Autodesk Fusion 360 part; units mm, degrees
sketch "Sketch1" plane through (0, 0, 0) normal (0, 0, 1) x (1, 0, 0)
  line L0 (0, 0) -> (26, 0)
  line L1 (26, 0) -> (26, 35.8)
  line L2 (26, 35.8) -> (0, 35.8)
  line L3 (0, 35.8) -> (0, 0)
  circle A0 centre (23.75, 30.8) radius 1.5
  circle A1 centre (2.25, 30.8) radius 1.5
  circle A2 centre (2.25, 4.8) radius 1.5
  circle A3 centre (23.75, 4.8) radius 1.5
  circle A4 centre (13, 25.8) radius 3.5
  line L4 (21.5, 27.2) -> (20.2, 27.2)
  line L5 (20.2, 27.2) -> (20.2, 24.4)
  line L6 (20.2, 24.4) -> (21.5, 24.4)
  line L7 (21.5, 24.4) -> (21.5, 27.2)
  dimension "d1" = 26
  dimension "d2" = 35.8
  dimension "d3" = 3
  dimension "d4" = 3
  dimension "d5" = 3
  dimension "d6" = 3
  dimension "d7" = 5
  dimension "d10" = 31
  dimension "d11" = 31
  dimension "d12" = 5
  dimension "d13" = 2.25
  dimension "d14" = 2.25
  dimension "d15" = 2.25
  dimension "d16" = 2.25
  dimension "d17" = 7
  dimension "d18" = 10
  dimension "d21" = 1.3
  dimension "d22" = 2.8
  dimension "d23" = 13
  dimension "d24" = 7.2
  dimension "d25" = 8.6
extrude "Extrude1" add sketch "Sketch1" along normal blind 2
Read the model definition and answer for the solid it produces. Units are mm, in the model's axes. A direction names the side the tool comes from. Coordinates: 2 decimals unless noted, no trailing zeros. Order: outer loops, then holes, each group sorted by start corner. A loop starts at its lowest first (then second) coordinate and runs counter-clockwise, first axis right, second up. Notation, with made-up numbers: (5.5, -21.75) -> (32.5, -21.75) arc R33 cw to (32.5, 9.25) -> close; hole circle Ø1 at (66, 1). An arc over 180 degrees is marked (long way). Answer as a JSON object with one key per item and string values.
1) The mould has two halves that part along Y. Classify faces 1 (the face through (1.925, 32.264, 0.986)), 2 (the face through (13, 35.8, 1)), 3 (the face through (23.425, 32.264, 0.986)), 4 (the face through (0, 18, 1)): released by +Y, released by -Y, zero draft, split by the parting line, or undercut.
Model answer:
{"face 1": "undercut", "face 2": "released by +Y", "face 3": "undercut", "face 4": "zero draft"}
2) A cutting plane is placed at A-A, the plane y = 4.8. Determine the outline of the cut face in (x, z).
Model answer:
{"outline": "(0, 0) -> (0.75, 0) -> (0.75, 2) -> (0, 2) -> close; (3.75, 0) -> (22.25, 0) -> (22.25, 2) -> (3.75, 2) -> close; (25.25, 0) -> (26, 0) -> (26, 2) -> (25.25, 2) -> close"}
3) A cutting plane is placed at D-D, the plane x = 13. Determine the outline of the cut face in (y, z), plus the area to 3 significant figures.
Model answer:
{"outline": "(0, 0) -> (22.3, 0) -> (22.3, 2) -> (0, 2) -> close; (29.3, 0) -> (35.8, 0) -> (35.8, 2) -> (29.3, 2) -> close", "area": "57.6 mm²"}
4) A cutting plane is placed at C-C, the plane z = 0.5. Determine the outline of the cut face in (x, y).
Model answer:
{"outline": "(0, 0) -> (26, 0) -> (26, 35.8) -> (0, 35.8) -> close; hole circle Ø3 at (2.25, 4.8); hole circle Ø3 at (2.25, 30.8); hole circle Ø7 at (13, 25.8); hole (20.2, 24.4) -> (21.5, 24.4) -> (21.5, 27.2) -> (20.2, 27.2) -> close; hole circle Ø3 at (23.75, 4.8); hole circle Ø3 at (23.75, 30.8)"}
5) Consider line 1 along Y through (x, z) = (23.75, 1.25); line 2 along Y through (x, z) = (22.5, 1.6); line 3 along X through (y, z) = (6, 1.15). Determine where each line is inside the solid, lowest interval first. Write a range as from..to.
Model answer:
{"line 1": "y = 0..3.3, 6.3..29.3, 32.3..35.8", "line 2": "y = 0..3.97, 5.63..29.97, 31.63..35.8", "line 3": "x = 0..1.35, 3.15..22.85, 24.65..26"}
6) A tool of negligible diameter and unlimited length cuts with its end or side. For faces 5 (the face through (13, 0, 1)), 6 (the face through (20.2, 26, 1)), from which of +Z, -Z, +X, -X, +Y, -Y can it reach the whole face along a straight path? Write none if from no direction.
Model answer:
{"face 5": "+Z, -Z, +X, -X, -Y", "face 6": "+Z, -Z"}
7) A cutting plane is placed at B-B, the plane x = 23.75. Determine the outline of the cut face in (y, z).
Model answer:
{"outline": "(0, 0) -> (3.3, 0) -> (3.3, 2) -> (0, 2) -> close; (6.3, 0) -> (29.3, 0) -> (29.3, 2) -> (6.3, 2) -> close; (32.3, 0) -> (35.8, 0) -> (35.8, 2) -> (32.3, 2) -> close"}
8) This flat-tipped pin is pushed along its axis until it touches: pin 1 (2.5 mm diameter, centred on x = 2.25, y = 30.8, fed in from -Z). Where does it stop, or does it pass through?
Model answer:
{"pin 1": "passes through"}
